Work out the finished part from the listing and answer in its coordinate system (mm). Round coordinates to 2 decimals unless told otherwise and drop trailing zeros. Order: outer loops, then holes, each group sorted by start corner. A loop starts at its lowest first (then second) coordinate and runs counter-clockwise, first axis right, second up. Notation, with made-up numbers: (18, 83.25) - (23, 83.25) arc R24 cw to (23, 96.25) - close; hole circle Ø7 at (13.5, 29.5). An arc over 180 degrees is marked (long way). Use CSV: the item, a comma, the result in double quotes.
from build123d import *

# Parameters (mm, degrees)
F1_DEPTH      = 1
F1_DEPTH_BACK = 1
F2_R          = 5


with BuildPart() as f1:
    # F0 (on Front) → F1 (new body, two sides)
    with BuildSketch(Plane.XZ) as f1_sk:
        Polygon((1, 55), (-1, 55), (-1, 67), (-3, 67), (-3, 80), (-1, 80), (-1, 110), (-4, 110), (-4, 65), (-7, 65), (-7, 15), (-60, 4.999998), (-60, 0), (60, 0), (60, 5), (7, 15), (7, 65), (4, 65), (4, 110), (1, 110), (1, 80), (3, 80), (3, 67), (1, 67), align=None)
    extrude(amount=F1_DEPTH)
    extrude(f1_sk.sketch, amount=-F1_DEPTH_BACK)

    # F2
    f2_edges = [f1.edges().sort_by_distance(p)[0] for p in [
        (-60, 0, 4.999998),
        (60, 0, 5),
    ]]
    fillet(f2_edges, radius=F2_R)


solid = f1.part
(1) Find section C-C (z = 69). Determine the outline of the cut face in (x, y).
Findings below:
outline,"(-4, -1) - (-3, -1) - (-3, 1) - (-4, 1) - close; (3, -1) - (4, -1) - (4, 1) - (3, 1) - close"
(2) Find section A-A (z = 84.5). Determine the outline of the cut face in (x, y), and give its area (3 significant figures).
Findings below:
outline,"(-4, -1) - (-1, -1) - (-1, 1) - (-4, 1) - close; (1, -1) - (4, -1) - (4, 1) - (1, 1) - close"
area,"12.0 mm²"
(3) Find the intervals of material crossed by L1, parallel to X at y = -0.55, z = 88; L2, parallel to Z at x = 2, y = 0.1; L3, parallel to X at y = -0.85, z = 63, in increasing order. Write a range as from..to.
Findings below:
L1,"x = -4..-1, 1..4"
L2,"z = 0..67, 80..110"
L3,"x = -7..-1, 1..7"
(4) Find section B-B (y = 0.7). Determine the outline of the cut face in (x, z).
Findings below:
outline,"(-60, 0) - (60, 0) - (60, 0.86) arc R5 ccw to (55.93, 5.77) - (7, 15) - (7, 65) - (4, 65) - (4, 110) - (1, 110) - (1, 80) - (3, 80) - (3, 67) - (1, 67) - (1, 55) - (-1, 55) - (-1, 67) - (-3, 67) - (-3, 80) - (-1, 80) - (-1, 110) - (-4, 110) - (-4, 65) - (-7, 65) - (-7, 15) - (-55.93, 5.77) arc R5 ccw to (-60, 0.86) - close"
(5) Each of these flat-tipped pins is pushed along its axis until it touches: pin 1 (1 mm diameter, centred on y = 0, z = 94.5, fed in from +X); pin 2 (0.6 mm diameter, centred on y = -0.5, z = 75, fed in from -X); pin 3 (1 mm diameter, centred on x = 5, y = -0.5, fed in from +Z). Where does it stop, or does it pass through?
Findings below:
pin 1,"stops at x = 4"
pin 2,"stops at x = -4"
pin 3,"stops at z = 65"
(6) Find section D-D (z = 50). Determine the outline of the cut face in (x, y), and give its area (3 significant figures).
Findings below:
outline,"(-7, -1) - (7, -1) - (7, 1) - (-7, 1) - close"
area,"28.0 mm²"
